from build123d import *

# Parameters (mm, degrees)
SKETCH1_W           = 71
SKETCH1_H           = 71
SKETCH1_R           = 2
SKETCH1_R_2         = 17.5
BOSS_EXTRUDE1_DEPTH = 3
FILLET2_R           = 8
SKETCH2_R           = 31
SKETCH2_R_2         = 30.5
CUT_EXTRUDE1_DEPTH  = 2
FILLET3_R           = 5
FILLET4_R           = 3
FILLET5_R           = 1
SKETCH4_R           = 32.5
SKETCH4_R_2         = 2
SKETCH4_R_3         = 29
SKETCH4_R_4         = 17.5
CUT_EXTRUDE4_DEPTH  = 2
FILLET8_R           = 4
FILLET9_R           = 4


with BuildPart() as part:
    # Sketch1 → Boss-Extrude1 (new body)
    with BuildSketch(Plane(origin=(0, 0, 0), x_dir=(1, 0, 0), z_dir=(0, 1, 0))):
        with Locations((35.5, 35.5)):
            Rectangle(SKETCH1_W, SKETCH1_H)
        with Locations(Location((6, 6, 0), (0, 0, 270))):
            Circle(SKETCH1_R, mode=Mode.SUBTRACT)
        with Locations(Location((65, 6, 0), (0, 0, 270))):
            Circle(SKETCH1_R, mode=Mode.SUBTRACT)
        with Locations(Location((65, 65, 0), (0, 0, 270))):
            Circle(SKETCH1_R, mode=Mode.SUBTRACT)
        with Locations(Location((6, 65, 0), (0, 0, 270))):
            Circle(SKETCH1_R, mode=Mode.SUBTRACT)
        with Locations(Location((35.5, 35.5, 0), (0, 0, 270))):
            Circle(SKETCH1_R_2, mode=Mode.SUBTRACT)
    extrude(amount=BOSS_EXTRUDE1_DEPTH)

    # Fillet2
    fillet2_edges = [part.edges().sort_by_distance(p)[0] for p in [
        (0, 1.5, -71),
        (71, 1.5, -71),
        (71, 1.5, 0),
        (0, 1.5, 0),
    ]]
    fillet(fillet2_edges, radius=FILLET2_R)

    # Sketch2 → Cut-Extrude1 (cut)
    with BuildSketch(Plane(origin=(0, 3, 0), x_dir=(1, 0, 0), z_dir=(0, 1, 0))):
        with Locations(Location((35.5, 35.5, 0), (0, 0, 270))):
            Circle(SKETCH2_R)
        with Locations(Location((35.5, 35.5, 0), (0, 0, 270))):
            Circle(SKETCH2_R_2, mode=Mode.SUBTRACT)
    extrude(amount=-CUT_EXTRUDE1_DEPTH, mode=Mode.SUBTRACT)

    # Fillet3
    # the kernel refuses this fillet: 5 mm, written as the material it takes off along each edge
    with BuildSketch(Plane(origin=(35.5, 3, -35.5), x_dir=(0, 0, 1), z_dir=(-1, 0, 0))) as fillet3_piece_1:
        with BuildLine():
            CenterArc((26.5, -5), FILLET3_R, 36.869897646, 53.130102354)
            Line((30.5, -2), (30.58, -1.94))
            ThreePointArc((30.58, -1.94), (30.6, -1), (30.6, 0))
            Line((30.6, 0), (30.5, 0.1))
            Line((30.5, 0.1), (26.5, 0.1))
            Line((26.5, 0.1), (26.5, 0))
        make_face()
    revolve(axis=Axis((35.5, 3, -35.5), (0, 1, 0)), mode=Mode.SUBTRACT)

    # Fillet4
    # the kernel refuses this fillet: 3 mm, written as the material it takes off along each edge
    with BuildSketch(Plane(origin=(35.5, 3, -35.5), x_dir=(0, 0, 1), z_dir=(-1, 0, 0))) as fillet4_piece_1:
        with BuildLine():
            CenterArc((33.828427125, -3), FILLET4_R, 90, 70.528779366)
            Line((31, -2), (30.943431458, -1.98))
            ThreePointArc((30.943431458, -1.98), (30.94, -1), (30.94, 0))
            Line((30.94, 0), (31, 0.06))
            Line((31, 0.06), (33.828427125, 0.06))
            Line((33.828427125, 0.06), (33.828427125, 0))
        make_face()
    revolve(axis=Axis((35.5, 3, -35.5), (0, 1, 0)), mode=Mode.SUBTRACT)

    # Fillet5
    fillet5_edges = [part.edges().sort_by_distance(p)[0] for p in [
        (35.5, 3, -53),
    ]]
    fillet(fillet5_edges, radius=FILLET5_R)

    # Sketch4 → Cut-Extrude4 (cut)
    # profile 1 of 2: a face of its own
    with BuildSketch(Plane(origin=(0, 0, 0), x_dir=(-1, 0, 0), z_dir=(0, -1, 0))):
        with BuildLine():
            ThreePointArc((-8, 0), (-2.343145751, 2.343145751), (0, 8))
            Line((0, 8), (0, 63))
            ThreePointArc((0, 63), (-2.343145751, 68.656854249), (-8, 71))
            Line((-8, 71), (-63, 71))
            ThreePointArc((-63, 71), (-68.656854249, 68.656854249), (-71, 63))
            Line((-71, 63), (-71, 8))
            ThreePointArc((-71, 8), (-68.656854249, 2.343145751), (-63, 0))
            Line((-63, 0), (-8, 0))
        make_face()
        with Locations(Location((-35.5, 35.5, 0), (0, 0, 90))):
            Circle(SKETCH4_R, mode=Mode.SUBTRACT)
        with Locations(Location((-6, 6, 0), (0, 0, 90))):
            Circle(SKETCH4_R_2, mode=Mode.SUBTRACT)
        with Locations(Location((-6, 65, 0), (0, 0, 90))):
            Circle(SKETCH4_R_2, mode=Mode.SUBTRACT)
        with Locations(Location((-65, 6, 0), (0, 0, 90))):
            Circle(SKETCH4_R_2, mode=Mode.SUBTRACT)
        with Locations(Location((-65, 65, 0), (0, 0, 90))):
            Circle(SKETCH4_R_2, mode=Mode.SUBTRACT)
    # profile 2 of 2: a face of its own
    with BuildSketch(Plane(origin=(0, 0, 0), x_dir=(-1, 0, 0), z_dir=(0, -1, 0))):
        with Locations(Location((-35.5, 35.5, 0), (0, 0, 90))):
            Circle(SKETCH4_R_3)
        with Locations((-35.5, 35.5)):
            Circle(SKETCH4_R_4, mode=Mode.SUBTRACT)
    extrude(amount=-CUT_EXTRUDE4_DEPTH, mode=Mode.SUBTRACT)

    # Fillet8
    # the kernel refuses this fillet: 4 mm, written as the material it adds along each edge
    with BuildSketch(Plane(origin=(35.5, 2, -35.5), x_dir=(0, 0, -1), z_dir=(-1, 0, 0))) as fillet8_piece_1:
        with BuildLine():
            CenterArc((25.535898385, 4), FILLET8_R, 270, 60)
            Line((25.535898385, 0), (25.535898385, -0.08))
            Line((25.535898385, -0.08), (29, -0.08))
            Line((29, -0.08), (29.08, 0))
            ThreePointArc((29.08, 0), (29.08, 1), (29.069282032, 1.96))
            Line((29.069282032, 1.96), (29, 2))
        make_face()
    revolve(axis=Axis((35.5, 2, -35.5), (0, -1, 0)))

    # Fillet9
    # the kernel refuses this fillet: 4 mm, written as the material it adds along each edge
    with BuildSketch(Plane(origin=(35.5, 2, -35.5), x_dir=(0, 0, -1), z_dir=(-1, 0, 0))) as fillet9_piece_1_section:
        with BuildLine():
            CenterArc((35.964101615, 4), FILLET9_R, 210, 60)
            Line((35.964101615, 0), (35.964101615, -0.08))
            Line((35.964101615, -0.08), (32.5, -0.08))
            Line((32.5, -0.08), (32.42, 0))
            ThreePointArc((32.42, 0), (32.42, 1), (32.430717968, 1.96))
            Line((32.430717968, 1.96), (32.5, 2))
        make_face()
    fillet9_piece_1 = revolve(axis=Axis((35.5, 2, -35.5), (0, -1, 0)), mode=Mode.PRIVATE)
    fillet9_piece_1 = split(fillet9_piece_1, bisect_by=Plane(origin=(35.5, 1.533400125, 0), z_dir=(0, 0, -1)), keep=Keep.TOP, mode=Mode.PRIVATE)
    fillet9_piece_1 = split(fillet9_piece_1, bisect_by=Plane(origin=(0, 1.533400125, -1.575907898), z_dir=(1, 0, 0)), keep=Keep.TOP, mode=Mode.PRIVATE)
    fillet9_piece_1 = split(fillet9_piece_1, bisect_by=Plane(origin=(35.5, 1.533400125, -71), z_dir=(0, 0, 1)), keep=Keep.TOP, mode=Mode.PRIVATE)
    fillet9_piece_1 = split(fillet9_piece_1, bisect_by=Plane(origin=(71, 1.533400125, -1.575907898), z_dir=(-1, 0, 0)), keep=Keep.TOP, mode=Mode.PRIVATE)
    add(fillet9_piece_1)


solid = part.part
Part model, mm, in its own coordinate system. A direction names the side the tool comes from. Give positions to 0.01 mm unless a question says otherwise; leave off trailing zeros. Loops run counter-clockwise (first coordinate to the right, second up) from the corner with the lowest first, then second, coordinate; pieces in that order, holes last.
(1) Pull direction Z, two halves, no side cores. Call faces 1 (the flat face through (63, 2, -7)), 2 (the cylindrical face through (7.352, 2.493, -7.474)), 3 (the cylindrical face through (2.281, 2.507, -2.406)): pulls with the +Z half, pulls with the -Z half, needs draft (parallel to the pull), parting line crosses it, or undercut.
Return value:
face 1: needs draft
face 2: undercut
face 3: pulls with the +Z half
(2) Pin check, flat tips, straight feed: pin 1 (2.5 mm diameter, centred on x = 6, z = -6, fed in from +Y); pin 2 (8 mm diameter, centred on x = 48.5, z = -44, fed in from +Y); pin 3 (1 mm diameter, centred on x = 41.5, y = 1, fed in from -Z). Stop position of each tip, or through.
Return value:
pin 1: passes through
pin 2: stops at y = 3
pin 3: stops at z = -69
(3) Band-saw the part on A-A (y = 0.5). Write the cut outline in (x, z), and give its area (3 significant figures).
Return value:
outline: circle Ø65.68 at (35.5, -35.5); hole circle Ø57.32 at (35.5, -35.5)
area: 808 mm2
(4) 3-axis set-ups, long thin cutter, end or side, ignore diameter. For faces 4 (the flat face through (8, 2, -63)), 5 (the flat face through (64, 2, -63)), 6 (the flat face through (15, 1, -12.7)): which of +Z, -Z, +X, -X, +Y, -Y reach the whole face in a straight line?
Return value:
face 4: -Z, -X, -Y
face 5: -Z, +X, -Y
face 6: +Y
(5) Drill centre lines: line 1 along Z through (x, y) = (48, 1.2); line 2 along Y through (x, z) = (57.5, -6.5); line 3 along X through (y, z) = (2.05, -30). Where is each one in solid material? Low to high.
Return value:
line 1: z = -66.65 to -63.95, -63.15 to -60.48, -10.52 to -7.85, -7.05 to -4.35
line 2: y = 2 to 3
line 3: x = 0 to 4.34, 6.59 to 18.89, 52.11 to 64.41, 66.66 to 71
